Autodesk Inventor part; units mm, degrees
ref_plane "YZ Plane" through (0, 0, 0) normal (1, 0, 0) x (0, 1, 0)
ref_plane "XZ Plane" through (0, 0, 0) normal (0, 1, 0) x (-1, 0, 0)
ref_plane "XY Plane" through (0, 0, 0) normal (0, 0, 1) x (1, 0, 0)
ref_plane "Work Plane1" through (60.6116, 29.9097, 55) normal (0, 0, 1) x (1, 0, 0)
sketch "Sketch1" plane through (60.6116, 29.9097, 55) normal (0, 0, 1) x (1, 0, 0)
  circle A0 centre (-11.75, -9.4206) radius 1.5
  circle A1 centre (-6.6055, -15.5471) radius 1.5
  arc A2 (-9.4525, -7.4914) -> (-14.0475, -11.3498) centre (-11.75, -9.4206) ccw
  arc A3 (-8.903, -17.4763) -> (-4.3081, -13.618) centre (-6.6055, -15.5471) ccw
  line L0 (-9.4525, -7.4914) -> (-4.3081, -13.618)
  line L1 (-8.903, -17.4763) -> (-14.0475, -11.3498)
  line L2 (-11.489, -10.8977) -> (-8.0153, -15.0346)
  line L3 (-10.3403, -9.9331) -> (-6.8665, -14.07)
  line L4 (-11.75, -9.4206) -> (-6.6055, -15.5471) construction
  point P0 (-60.6116, -29.9097)
  dimension "d0" = 6
  dimension "d1" = 6
  dimension "d2" = 1.5
extrude "Extrusion1" add sketch "Sketch1" along normal blind 4
sketch "Sketch2" plane through (51.7087, 12.4334, 55) normal (-0.7658175, -0.643058, 0) x (0, 0, 1)
  line L0 (4, 0) -> (4, 8)
  line L1 (4, 4) -> (0, 4) construction
  line L2 (0, 6.701) -> (0, 1.299)
  line L3 (0, 0) -> (4, 0)
  line L4 (2, 0) -> (2, 8) construction
  line L5 (0, 8) -> (4, 8)
  point P0 (-55, 23.7299)
  point P1 (2, 4)
hole "Hole1" at (49.1364, 15.4967, 57) direction (0.7658175, 0.643058, 0) diameter 2.4 end through all
properties part number "rail_holder"
Can you work these out from the model? Positions are in its coordinate system, mm. A direction names the side the tool comes from. Round coordinates to 2 decimals unless told otherwise and drop trailing zeros. Loops run counter-clockwise (first coordinate to the right, second up) from the corner with the lowest first, then second, coordinate; pieces in that order, holes last.
Item 1: Will this pin go through, and if not, where does the flat tip stop? pin 1 Ø2 at (x, z) = (53.5, 56) entering from +Y.
Item 2: Suppose I cut it at C-C, the plane x = 55. Write out the boundary of the cut face in (y, z).
Item 3: Suppose I cut it at B-B, the plane y = 21. Write out the boundary of the cut face in (x, z), then the cut area to 3 significant figures.
Item 4: Which directions (+Z, -Z, +X, -X, +Y, -Y) give clear straight access to the entire face, cutting with the end or side of a thin tool? Please do faces 1 (the flat face through (53.695, 19.398, 55.639)), 2 (the flat face through (50.835, 16.973, 55.639)).
Item 5: If we mould it in two halves opening along Y, with no side actions, what happens to faces 3 (the cylindrical face through (55.99, 12.11, 56.97)), 4 (the flat face through (50.1, 17.5, 59)), 5 (the flat face through (49.172, 15.454, 55.639)), 6 (the cylindrical face through (50.31, 15.88, 55.89))? For each: +Y half, -Y half, draft (parallel to the pull), parting line (faces both ways), or undercut.
Item 6: Suppose I cut it at A-A, the plane z = 57.4. Write out the boundary of the cut face in (x, y), then the cut area to 3 significant figures.
Item 7: Suppose I cut it at D-D, the plane z = 56.45. Write out the boundary of the cut face in (x, y), then the cut area to 3 significant figures.
Item 8: Please list where these lines run through material, in increasing order: L1, parallel to X at y = 20.75, z = 56.6; L2, parallel to X at y = 20.5, z = 58.85; L3, parallel to Y at x = 51, z = 58.55.
Reported:
1. pin 1: stops at y = 20.82
2. outline: (11.53, 55) - (13.24, 55) - (13.24, 59) - (11.53, 59) - close; (15.49, 55) - (17.84, 55) - (17.84, 59) - (15.49, 59) - close
3. outline: (45.91, 55) - (47.45, 55) - (47.45, 59) - (45.91, 59) - close; (50.27, 55) - (52.35, 55) - (52.35, 59) - (50.27, 59) - close
3. area: 14.5 mm2
4. face 1: +Z, -Z, +X, +Y
4. face 2: +Z, -Z
5. face 3: parting line
5. face 4: draft
5. face 5: -Y half
5. face 6: undercut
6. outline: (46.56, 18.56) - (48.41, 16.36) - (50.13, 17.81) - (49.12, 19.01) arc R1.5 cw (long way) to (50.27, 19.98) - (51.28, 18.77) - (53, 20.22) - (51.16, 22.42) arc R3 ccw to start; (49.86, 14.63) - (51.71, 12.43) arc R3 ccw to (56.3, 16.29) - (54.46, 18.49) - (52.74, 17.04) - (53.75, 15.84) arc R1.5 cw (long way) to (52.6, 14.88) - (51.59, 16.08) - close
6. area: 44.3 mm2
7. outline: (46.56, 18.56) - (48.45, 16.31) - (50.17, 17.76) - (49.12, 19.01) arc R1.5 cw (long way) to (50.27, 19.98) - (51.32, 18.72) - (53.05, 20.17) - (51.16, 22.42) arc R3 ccw to start; (49.82, 14.68) - (51.71, 12.43) arc R3 ccw to (56.3, 16.29) - (54.42, 18.54) - (52.69, 17.09) - (53.75, 15.84) arc R1.5 cw (long way) to (52.6, 14.88) - (51.55, 16.13) - close
7. area: 44.8 mm2
8. L1: x = 45.87 to 47.38, 50.34 to 52.56
8. L2: x = 45.86 to 47.36, 50.36 to 52.77
8. L3: y = 13.28 to 16.78, 19.11 to 22.59
